Check sheet for the modelled part. Datum: model origin and axes. Units: mm. A direction names the side the tool comes from. Round coordinates to 2 decimals unless told otherwise and drop trailing zeros. Write each loop counter-clockwise with the first axis right and the second up, starting at its lowest first coordinate (ties: lowest second). Pieces come first, ordered by that corner, then holes.
Item 1: Tool access check on faces 4 (the flat face through (-1, 50, 2)), 5 (the cylindrical face through (-0.59, 14.46, 4.01)). Record the directions out of +Z, -Z, +X, -X, +Y, -Y that give a thin tool (end or side, any length) a straight path to the whole face; none if there is none.
Item 2: Material ranges on line 1 (Y direction, x = -40, z = 2.8) (3 decimals); line 2 (Y direction, x = -20, z = 1.8) (3 decimals); line 3 (Y direction, x = -10, z = 3.75), recorded low to high.
Item 3: Go/stop test with a flat-tipped pin: pin 1 Ø2.5 at (x, y) = (-1.5, -8) entering from +Z. Record where the tip stops, or that it passes through.
Item 4: Cross-section at B-B on z = 4. Count the separate pieces of the cut face and the enclosed holes in it, plus the area to 4 significant figures.
Item 5: Cross-section at A-A on x = 0. Enter the section's corners in (y, z) (3 decimals).
Item 6: Cross-section at D-D on x = -20. Enter the section's corners in (y, z) (3 decimals), plus the area to 3 significant figures.
Item 7: Cross-section at C-C on x = 10. Enter the section's corners in (y, z).
Item 8: Release check for a two-part mould opening along X. For faces 1 (the cylindrical face through (46.99, -52.15, 2.54)), 2 (the cylindrical face through (-37.5, 0.8, 2.5)), 3 (the flat face through (-1, -2, 0)) record: +X half, -X half, draft (parallel to the pull), parting line (faces both ways), or undercut.
from build123d import *

# Parameters (mm, degrees)
SKETCH_W        = 100
SKETCH_H        = 105
PAD_DEPTH       = 5
SKETCH001_R     = 4.5
POCKET_DEPTH    = 2
SKETCH002_R     = 2.5
POCKET001_DEPTH = 3
SKETCH003_R     = 2.625
POCKET002_DEPTH = 5
FILLET_R        = 10


with BuildPart() as part:
    # Sketch → Pad (new body)
    with BuildSketch(Plane.XY):
        with Locations((0, -2.5)):
            Rectangle(SKETCH_W, SKETCH_H)
    extrude(amount=PAD_DEPTH)

    # Sketch001 (on Face6 of Pad) → Pocket (cut)
    with BuildSketch(Plane.XY.offset(5)):
        with Locations((0, 10)):
            Circle(SKETCH001_R)
        with Locations((10, 0)):
            Circle(SKETCH001_R)
        with Locations((-10, 0)):
            Circle(SKETCH001_R)
        with Locations((0, -10)):
            Circle(SKETCH001_R)
    extrude(amount=-POCKET_DEPTH, mode=Mode.SUBTRACT)

    # Sketch002 (on Face4 of Pocket) → Pocket001 (cut)
    with BuildSketch(Plane(origin=(0, 0, 0), x_dir=(1, 0, 0), z_dir=(0, 0, -1))):
        with Locations((0, 10)):
            Circle(SKETCH002_R)
        with Locations((10, 0)):
            Circle(SKETCH002_R)
        with Locations((0, -10)):
            Circle(SKETCH002_R)
        with Locations((-10, 0)):
            Circle(SKETCH002_R)
    extrude(amount=-POCKET001_DEPTH, mode=Mode.SUBTRACT)

    # Sketch003 (on Face5 of Pocket001) → Pocket002 (cut)
    with BuildSketch(Plane.XY.offset(5)):
        with Locations((-40, 0)):
            Circle(SKETCH003_R)
        with Locations((-40, -20)):
            Circle(SKETCH003_R)
        with Locations((-20, -45)):
            Circle(SKETCH003_R)
        with Locations((20, -45)):
            Circle(SKETCH003_R)
        with Locations((40, -20)):
            Circle(SKETCH003_R)
        with Locations((40, 0)):
            Circle(SKETCH003_R)
        with Locations((40, 20)):
            Circle(SKETCH003_R)
        with Locations((40, 40)):
            Circle(SKETCH003_R)
        with Locations((20, 40)):
            Circle(SKETCH003_R)
        with Locations((0, 40)):
            Circle(SKETCH003_R)
        with Locations((-20, 40)):
            Circle(SKETCH003_R)
        with Locations((-40, 40)):
            Circle(SKETCH003_R)
        with Locations((-40, 20)):
            Circle(SKETCH003_R)
        with Locations((-20, -20)):
            Circle(SKETCH003_R)
        with Locations((20, -20)):
            Circle(SKETCH003_R)
    extrude(amount=-POCKET002_DEPTH, mode=Mode.SUBTRACT)

    # Fillet
    fillet_edges = [part.edges().sort_by_distance(p)[0] for p in [
        (-50, 50, 2.5),
        (50, 50, 2.5),
        (50, -55, 2.5),
        (-50, -55, 2.5),
    ]]
    fillet(fillet_edges, radius=FILLET_R)


solid = part.part
Response values:
1. face 4: +Z, -Z, +X, -X, +Y
1. face 5: +Z
2. line 1: y = -55 to -22.625, -17.375 to -2.625, 2.625 to 17.375, 22.625 to 37.375, 42.625 to 50
2. line 2: y = -55 to -47.625, -42.375 to -22.625, -17.375 to 37.375, 42.625 to 50
2. line 3: y = -55 to -4.5, 4.5 to 50
3. pin 1: stops at z = 3
4. separate pieces: 1
4. enclosed holes: 19
4. area: 9,835 mm2
5. outline: (-55, 0) - (-12.5, 0) - (-12.5, 3) - (-14.5, 3) - (-14.5, 5) - (-55, 5) - close; (-7.5, 0) - (7.5, 0) - (7.5, 3) - (5.5, 3) - (5.5, 5) - (-5.5, 5) - (-5.5, 3) - (-7.5, 3) - close; (12.5, 0) - (37.375, 0) - (37.375, 5) - (14.5, 5) - (14.5, 3) - (12.5, 3) - close; (42.625, 0) - (50, 0) - (50, 5) - (42.625, 5) - close
6. outline: (-55, 0) - (-47.625, 0) - (-47.625, 5) - (-55, 5) - close; (-42.375, 0) - (-22.625, 0) - (-22.625, 5) - (-42.375, 5) - close; (-17.375, 0) - (37.375, 0) - (37.375, 5) - (-17.375, 5) - close; (42.625, 0) - (50, 0) - (50, 5) - (42.625, 5) - close
6. area: 446 mm2
7. outline: (-55, 0) - (-2.5, 0) - (-2.5, 3) - (-4.5, 3) - (-4.5, 5) - (-55, 5) - close; (2.5, 0) - (50, 0) - (50, 5) - (4.5, 5) - (4.5, 3) - (2.5, 3) - close
8. face 1: +X half
8. face 2: undercut
8. face 3: draft
